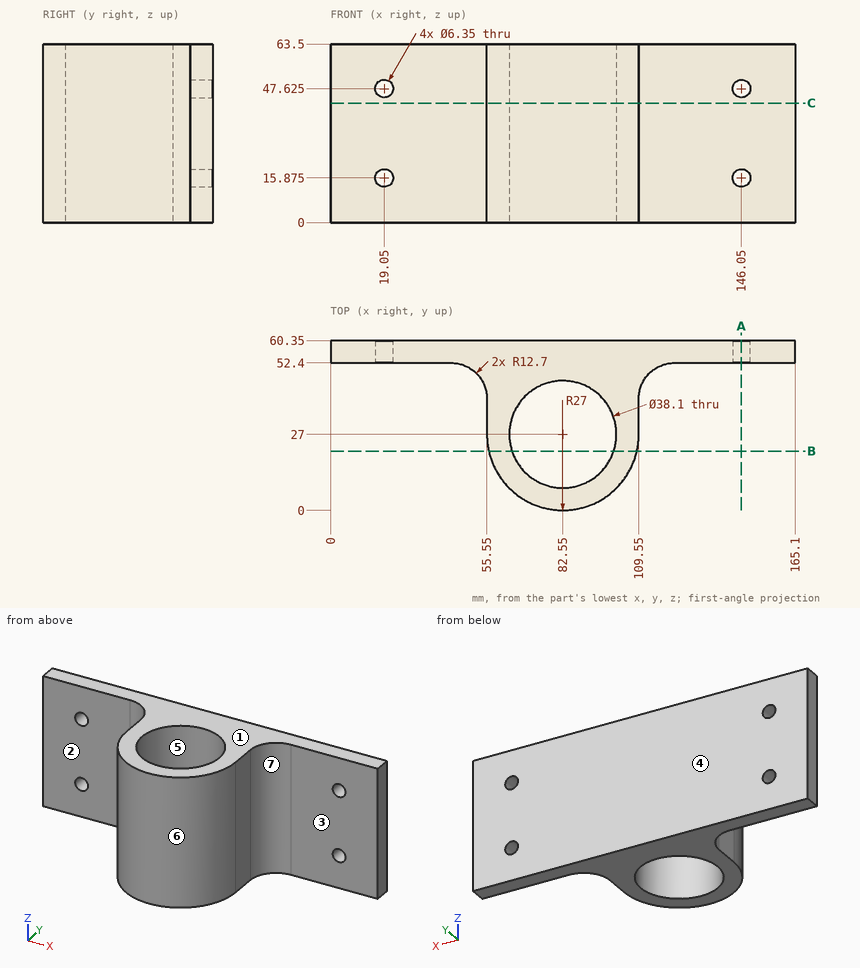
Design review of the part shown in the three views and the two pictorial views. Dimensions are in mm from the part's minimum x, y and z. A direction names the side the tool comes from. Round coordinates to 2 decimals unless told otherwise and drop trailing zeros. Write each loop counter-clockwise with the first axis right and the second up, starting at its lowest first coordinate (ties: lowest second). Pieces come first, ordered by that corner, then holes. Notation, with made-up numbers: (-37, -26) -> (-28, -26) arc R18 ccw to (-28, -13) -> close; hole circle Ø1 at (-3, 51.5). An arc over 180 degrees is marked (long way). Answer as a JSON object with one key per item and string values.
1. To check wall thickness, follow line 1 along Z through (x, y) = (19, 58); line 2 along X through (y, z) = (28, 57); line 3 along Y through (x, z) = (82.55, 25). State the ranges of each line that lie inside material, in increasing order.
Results found:
{"line 1": "z = 0 to 12.7, 19.05 to 44.45, 50.8 to 63.5", "line 2": "x = 55.55 to 63.53, 101.57 to 109.55", "line 3": "y = 0 to 7.95, 46.05 to 60.35"}
2. Clearance check with flat-ended pins moving along their axes: pin 1 (13 mm diameter, centred on x = 143.5, z = 16, fed in from -Y); pin 2 (5 mm diameter, centred on x = 19.05, z = 15.875, fed in from +Y); pin 3 (5 mm diameter, centred on y = 38.5, z = 44, fed in from -X); pin 4 (10 mm diameter, centred on y = 36.5, z = 16.5, fed in from -X). State where each tip first meets the part, or that it passes through.
Results found:
{"pin 1": "stops at y = 52.4", "pin 2": "passes through", "pin 3": "stops at x = 55.48", "pin 4": "stops at x = 55.42"}
3. We need section C-C on z = 42.5. State the section outline as (x, y) points.
Results found:
{"outline": "(0, 52.4) -> (42.85, 52.4) arc R12.7 cw to (55.55, 39.7) -> (55.55, 27) arc R27 ccw to (109.55, 27) -> (109.55, 39.7) arc R12.7 cw to (122.25, 52.4) -> (165.1, 52.4) -> (165.1, 60.35) -> (0, 60.35) -> close; hole circle Ø38.1 at (82.55, 27)"}
4. We need section A-A on x = 146.05. State the section outline as (y, z) points.
Results found:
{"outline": "(52.4, 0) -> (60.35, 0) -> (60.35, 12.7) -> (52.4, 12.7) -> close; (52.4, 19.05) -> (60.35, 19.05) -> (60.35, 44.45) -> (52.4, 44.45) -> close; (52.4, 50.8) -> (60.35, 50.8) -> (60.35, 63.5) -> (52.4, 63.5) -> close"}
5. We need section B-B on y = 21. State the section outline as (x, z) points (1 decimal), and give its area (3 significant figures).
Results found:
{"outline": "(56.2, 0) -> (64.5, 0) -> (64.5, 63.5) -> (56.2, 63.5) -> close; (100.6, 0) -> (108.9, 0) -> (108.9, 63.5) -> (100.6, 63.5) -> close", "area": "1,050 mm^2"}
6. Machinability: for the marked faces 1, 2 and 3, which of the approach directions +Z, -Z, +X, -X, +Y, -Y give a long, thin tool a straight path to every point of the face, cutting with its end or side? Answer none if there is none.
Results found:
{"face 1": "+Z, +X, -X, +Y, -Y", "face 2": "+Z, -Z, -X, -Y", "face 3": "+Z, -Z, +X, -Y"}
7. The part is to be moulded in two halves that separate along X. For the marked faces 4, 5, 6 and 7, say which applies: pulls with the +X half, pulls with the -X half, needs draft (parallel to the pull), parting line crosses it, or undercut.
Results found:
{"face 4": "needs draft", "face 5": "undercut", "face 6": "parting line crosses it", "face 7": "pulls with the +X half"}
